Autodesk Fusion 360 part; units mm, degrees
sketch "스케치1" plane through (0, 0, 0) normal (0, 1, 0) x (1, 0, 0)
  circle A0 centre (0, 0) radius 9
  circle A1 centre (0, 0) radius 2.5
  circle A2 centre (0, 0) radius 6 construction
  circle A3 centre (6, 0) radius 1
  circle A4 centre (4.2426, 4.2426) radius 1
  circle A5 centre (0, 6) radius 1
  circle A6 centre (-4.2426, 4.2426) radius 1
  circle A7 centre (-6, 0) radius 1
  circle A8 centre (-4.2426, -4.2426) radius 1
  circle A9 centre (0, -6) radius 1
  circle A10 centre (4.2426, -4.2426) radius 1
  circle A11 centre (0, 0) radius 1.15
  circle A12 centre (0, 0) radius 2.2
  circle A13 centre (0, 0) radius 3.5
  dimension "d1" = 18
  dimension "d2" = 5
  dimension "d3" = 12
  dimension "d4" = 2
  dimension "d6" = 360
  dimension "d7" = 2.3
  dimension "d10" = 4.4
  dimension "d11" = 7
extrude "돌출1" add sketch "스케치1" against normal blind 2 contours A0 | A1 | A12 | A13
extrude "돌출2" add sketch "스케치1" along normal blind 2.5 contours A1 | A13
Work out the finished part from the listing and answer in its coordinate system (mm). A direction names the side the tool comes from. Give positions to 0.01 mm unless a question says otherwise; leave off trailing zeros. Loops run counter-clockwise (first coordinate to the right, second up) from the corner with the lowest first, then second, coordinate; pieces in that order, holes last. Notation, with made-up numbers: (-20, -3) -> (32, -3) arc R17 ccw to (32, 23) -> close; hole circle Ø2 at (-22, 70). An arc over 180 degrees is marked (long way). One line per question, with ' | ' between items. Start each with the question number.
1) Determine the mould class of faces 1 (the face through (0, -2, 2)), 2 (the face through (0, -1, -7)), 3 (the face through (-1.172, -0.986, -8.923)) for opening direction X: +X half, -X half, draft (parallel to the pull), parting line (faces both ways), or undercut.
2) Section B-B, the plane x = 0 is taken. Determine the outline of the cut face in (y, z).
3) For faces 4 (the face through (4.78, -0.99, 3.4)), 5 (the face through (0, 0, 4)), determine the directions among +Z, -Z, +X, -X, +Y, -Y from which every point of the face is accessible in a straight line to the end or side of a thin tool.
4) Section A-A, the plane z = 0 is taken. Determine the outline of the cut face in (x, y), then the cut area to 3 significant figures.
5) Each of these flat-tipped pins is pushed along its axis until it touches: pin 1 (2 mm diameter, centred on x = 0.5, z = 0.5, fed in from +Y); pin 2 (2 mm diameter, centred on y = 0, z = -4.5, fed in from -X). Where does it stop, or does it pass through?
6) Straight lines are drawn through the part: L1, parallel to X at y = -0.45, z = 0; L2, parallel to X at y = -1.1, z = 3.75. For each, find the intervals that lie inside material, in ascending order.
7) Section C-C, the plane x = -6 is taken. Determine the outline of the cut face in (y, z).
8) Section D-D, the plane z = 6 is taken. Determine the outline of the cut face in (x, y).
Resolved:
1) face 1: draft | face 2: undercut | face 3: parting line
2) outline: (-2, -9) -> (0, -9) -> (0, -7) -> (-2, -7) -> close; (-2, -5) -> (0, -5) -> (0, -3.5) -> (2.5, -3.5) -> (2.5, -2.2) -> (0, -2.2) -> (0, -1.15) -> (-2, -1.15) -> close; (-2, 1.15) -> (0, 1.15) -> (0, 2.2) -> (2.5, 2.2) -> (2.5, 3.5) -> (0, 3.5) -> (0, 5) -> (-2, 5) -> close; (-2, 7) -> (0, 7) -> (0, 9) -> (-2, 9) -> close
3) face 4: +Y, -Y | face 5: +Y
4) outline: (-9, -2) -> (-7, -2) -> (-7, 0) -> (-9, 0) -> close; (-5, -2) -> (-1.15, -2) -> (-1.15, 0) -> (-2.2, 0) -> (-2.2, 2.5) -> (-3.5, 2.5) -> (-3.5, 0) -> (-5, 0) -> close; (1.15, -2) -> (5, -2) -> (5, 0) -> (3.5, 0) -> (3.5, 2.5) -> (2.2, 2.5) -> (2.2, 0) -> (1.15, 0) -> close; (7, -2) -> (9, -2) -> (9, 0) -> (7, 0) -> close | area: 29.9 mm2
5) pin 1: y = 0 | pin 2: x = -8.29
6) L1: -9 to -7, -5 to -1.15, 1.15 to 5, 7 to 9 | L2: -8.18 to -5.11, -3.37 to 3.37, 5.11 to 8.18
7) outline: (-2, -6.71) -> (0, -6.71) -> (0, -1) -> (-2, -1) -> close; (-2, 1) -> (0, 1) -> (0, 6.71) -> (-2, 6.71) -> close
8) outline: (-6.71, -2) -> (-1, -2) -> (-1, 0) -> (-6.71, 0) -> close; (1, -2) -> (6.71, -2) -> (6.71, 0) -> (1, 0) -> close
